```python
from build123d import *

# Parameters (mm, degrees)
CHAMFER1_SIZE  = 4.24981925
CHAMFER1_SIZE2 = 2.54


with BuildPart() as part:
    # Sketch1 → Revolve2 (revolve)
    with BuildSketch(Plane(origin=(0, 0, 0), x_dir=(0, 0, -1), z_dir=(1, 0, 0)), mode=Mode.PRIVATE) as revolve2_sk:
        Polygon((-1.6, 0), (-1.6, 5.231508424), (-25.4, 13.894), (-25.4, 15.494), (-1.6, 6.831508424), (-1.6, 15.494), (0, 15.494), (0, 0), align=None)
    revolve(revolve2_sk.sketch.rotate(Axis((0, 0, 1.6), (0, 0, -1)), 90), axis=Axis((0, 0, 1.6), (0, 0, -1)))  # turned: the seam where the file's is

    # Chamfer1
    chamfer1_edges = [part.edges().sort_by_distance(p)[0] for p in [
        (-5.231508424, 0, 1.6),
    ]]
    chamfer1_side = [part.faces().sort_by_distance(p)[0] for p in [
        (0, 0, 1.6),
    ]]
    chamfer(chamfer1_edges, length=CHAMFER1_SIZE, length2=CHAMFER1_SIZE2, reference=chamfer1_side[0])


solid = part.part
```
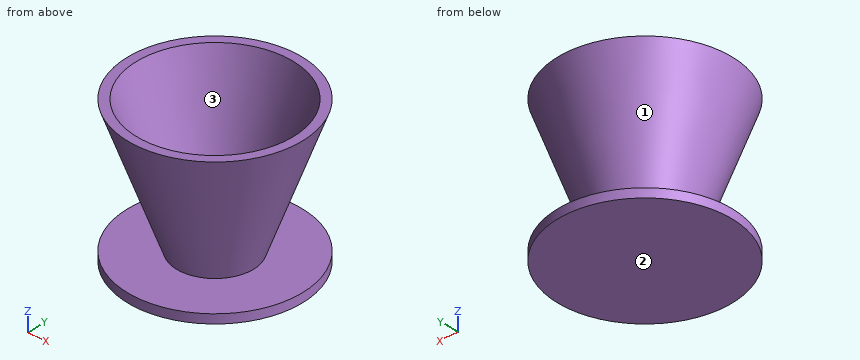
Design review of the part built by this model. Coordinates are the model's own, in mm. Face numbers are marked on the shaded views. Give positions to 0.01 mm unless a question says otherwise; leave off trailing zeros. Order: outer loops, then holes, each group sorted by start corner. A loop starts at its lowest first (then second) coordinate and runs counter-clockwise, first axis right, second up. Notation, with made-up numbers: (55.25, 13.25) -> (63.25, 13.25) arc R27 cw to (63.25, 30.25) -> close; hole circle Ø6 at (46, 61). An arc over 180 degrees is marked (long way). Write item = value, one per line. Start each with the question number.
(1) To check wall thickness, follow line 1 along Z through (x, y) = (5.5, 9.5); line 2 along X through (y, z) = (-2, 21.5); line 3 along Z through (x, y) = (-10, -10). State the ranges of each line that lie inside material, in increasing order.
(2) We need section D-D on z = 7.5. Write out the cut boundary in (x, y).
(3) Mouldability with a two-part tool opening along Z and no side actions: class the marked faces 1, 2 and 3 as +Z half, -Z half, draft (parallel to the pull), parting line (faces both ways), or undercut.
(4) We need section A-A on y = 0. Write out the cut boundary in (x, z), plus the area to 3 significant figures.
(5) We need section B-B on z = 23. Write out the cut boundary in (x, y).
(6) For pin 1 (3 mm diameter, centred on x = 0, z = 7.5, fed in from -Y); pin 2 (3 mm diameter, centred on x = 6.5, z = 4, fed in from +Y); pin 3 (10 mm diameter, centred on y = 6, z = 21, fed in from -X), all flat-tipped, find the tip position at first contact; note any pin that passes through.
Numbers:
q1.line_1 = 0 to 1.6, 12.99 to 17.39
q1.line_2 = -13.93 to -12.31, 12.31 to 13.93
q1.line_3 = 0 to 1.6, 21.69 to 25.4
q2.outline = circle Ø17.96 at (0, 0); hole circle Ø14.76 at (0, 0)
q3.face_1 = undercut
q3.face_2 = -Z half
q3.face_3 = +Z half
q4.outline = (-15.49, 0) -> (15.49, 0) -> (15.49, 1.6) -> (6.83, 1.6) -> (15.49, 25.4) -> (13.89, 25.4) -> (6.1, 3.99) -> (0.98, 1.6) -> (-0.98, 1.6) -> (-6.1, 3.99) -> (-13.89, 25.4) -> (-15.49, 25.4) -> (-6.83, 1.6) -> (-15.49, 1.6) -> close
q4.area = 136 mm^2
q5.outline = circle Ø29.24 at (0, 0); hole circle Ø26.04 at (0, 0)
q6.pin_1 = -9.52
q6.pin_2 = 6.05
q6.pin_3 = -15.07
